Design review of the part built by this model. Coordinates are the model's own, in mm. A direction names the side the tool comes from. Give positions to 0.01 mm unless a question says otherwise; leave off trailing zeros. Write each loop counter-clockwise with the first axis right and the second up, starting at its lowest first coordinate (ties: lowest second). Pieces come first, ordered by that corner, then holes. Notation, with made-up numbers: (31, -27) -> (84, -27) arc R24 ccw to (84, 12) -> close; hole circle Ø11 at (42, 11). An arc over 180 degrees is marked (long way). Use CSV: the item, a comma, the result in double quotes.
```python
from build123d import *

# Parameters (mm, degrees)
ESQUISSE1_R             = 7.5
EXTRUSION1_DEPTH        = 14
ESQUISSE2_R             = 9.75
EXTRUSION2_DEPTH        = 3
ESQUISSE3_R             = 6.5
EXTRUSION3_DEPTH        = 6.5
ESQUISSE4_R             = 4.5
ENL_V_MAT_EXTRU_1_DEPTH = 12.5
ENL_V_MAT_EXTRU_2_DEPTH = 5
CHANFREIN1_SIZE         = 1
CHANFREIN2_SIZE         = 0.3


with BuildPart() as part:
    # Esquisse1 → Extrusion1 (new body)
    with BuildSketch(Plane(origin=(0, 0, 0), x_dir=(1, 0, 0), z_dir=(0, 1, 0))):
        with Locations(Location((0, 0, 0), (0, 0, 270))):  # turned: the seam where the file's is
            Circle(ESQUISSE1_R)
    extrude(amount=-EXTRUSION1_DEPTH)

    # Esquisse2 → Extrusion2 (add)
    with BuildSketch(Plane(origin=(0, 0, 0), x_dir=(-1, 0, 0), z_dir=(0, 1, 0))):
        with Locations(Location((0, 0, 0), (0, 0, 90))):  # turned: the seam where the file's is
            Circle(ESQUISSE2_R)
    extrude(amount=EXTRUSION2_DEPTH)

    # Esquisse3 → Extrusion3 (add)
    with BuildSketch(Plane(origin=(0, 0, 0), x_dir=(1, 0, 0), z_dir=(0, 1, 0))):
        with Locations(Location((0, 0, 0), (0, 0, 270))):  # turned: the seam where the file's is
            Circle(ESQUISSE3_R)
    extrude(amount=EXTRUSION3_DEPTH)

    # Esquisse4 → Enlèv. mat.-Extru.1 (cut)
    with BuildSketch(Plane.XZ.offset(14)):
        with Locations(Location((0, 0, 0), (0, 0, 270))):  # turned: the seam where the file's is
            Circle(ESQUISSE4_R)
    extrude(amount=-ENL_V_MAT_EXTRU_1_DEPTH, mode=Mode.SUBTRACT)

    # Esquisse5 → Enlèv. mat.-Extru.2 (cut)
    with BuildSketch(Plane(origin=(0, 6.5, 0), x_dir=(-1, 0, 0), z_dir=(0, 1, 0))):
        Polygon((-4.618802154, 0), (-2.309401077, -4), (2.309401077, -4), (4.618802154, 0), (2.309401077, 4), (-2.309401077, 4), align=None)
    extrude(amount=-ENL_V_MAT_EXTRU_2_DEPTH, mode=Mode.SUBTRACT)

    # Chanfrein1
    chanfrein1_edges = [part.edges().sort_by_distance(p)[0] for p in [
        (0, -14, -7.5),
    ]]
    chamfer(chanfrein1_edges, length=CHANFREIN1_SIZE)

    # Chanfrein2
    chanfrein2_edges = [part.edges().sort_by_distance(p)[0] for p in [
        (0, 6.5, -6.5),
        (0, 0, -9.75),
        (0, 3, -9.75),
    ]]
    chamfer(chanfrein2_edges, length=CHANFREIN2_SIZE)


solid = part.part
```
(1) Take a section at B-B (x = 0). Write out the cut boundary in (y, z).
Established:
outline,"(-14, -6.5) -> (-13, -7.5) -> (0, -7.5) -> (0, -9.45) -> (0.3, -9.75) -> (2.7, -9.75) -> (3, -9.45) -> (3, -6.5) -> (6.2, -6.5) -> (6.5, -6.2) -> (6.5, -4) -> (1.5, -4) -> (1.5, 4) -> (6.5, 4) -> (6.5, 6.2) -> (6.2, 6.5) -> (3, 6.5) -> (3, 9.45) -> (2.7, 9.75) -> (0.3, 9.75) -> (0, 9.45) -> (0, 7.5) -> (-13, 7.5) -> (-14, 6.5) -> (-14, 4.5) -> (-1.5, 4.5) -> (-1.5, -4.5) -> (-14, -4.5) -> close"
(2) Clearance check with flat-ended pins moving along their axes: pin 1 (8 mm diameter, centred on x = -1, z = 0.5, fed in from -Y); pin 2 (5 mm diameter, centred on x = -7.5, z = -7, fed in from +Y); pin 3 (3 mm diameter, centred on x = -2.5, y = -6.5, fed in from -Z); pin 4 (1.5 mm diameter, centred on x = -6, y = -3, fed in from +Z). State where each tip first meets the part, or that it passes through.
Established:
pin 1,"stops at y = -14"
pin 2,"stops at y = 3"
pin 3,"stops at z = -7.43"
pin 4,"stops at z = 5.36"
(3) Tool access review of faces 5 (the face through (-3.48, 4.04, 1.97)), 6 (the face through (0.33, -6.409, -7.493)), 7 (the face through (9.667, 1.483, -1.269)): name each direction out of +Z, -Z, +X, -X, +Y, -Y from which nothing blocks a thin tool from reaching the whole face with its end or side.
Established:
face 5,"+Y"
face 6,"-Y"
face 7,"+Y, -Y"
(4) Take a section at A-A (y = 3.75). Write out the cut boundary in (x, z).
Established:
outline,"circle Ø13 at (0, 0); hole (-4.62, 0) -> (-2.31, -4) -> (2.31, -4) -> (4.62, 0) -> (2.31, 4) -> (-2.31, 4) -> close"
(5) Take a section at C-C (y = -8). Write out the cut boundary in (x, z).
Established:
outline,"circle Ø15 at (0, 0); hole circle Ø9 at (0, 0)"
(6) Mouldability with a two-part tool opening along Z and no side actions: class faces 1 (the face through (0, -1.5, 0)), 2 (the face through (-3.955, 4.578, -5.158)), 3 (the face through (-4.05, 6.5, 1.29)), 4 (the face through (1.352, -7.838, -4.292)) as +Z half, -Z half, draft (parallel to the pull), parting line (faces both ways), or undercut.
Established:
face 1,"undercut"
face 2,"parting line"
face 3,"draft"
face 4,"undercut"
(7) For line 1 along X through (y, z) = (-4.25, 0); line 2 along Y through (x, z) = (1, 0.75); line 3 along X through (y, z) = (5, 2), list the stretches that pass through material, from the lowest coordinate up. Write a range as [from, to].
Established:
line 1,"x = [-7.5, -4.5], [4.5, 7.5]"
line 2,"y = [-1.5, 1.5]"
line 3,"x = [-6.18, -3.46], [3.46, 6.18]"
